from build123d import *

# Parameters (mm, degrees)
F0_W     = 57.15
F0_H     = 38.1
F1_DEPTH = 6.35
F3_DEPTH = 19.05
F5_DEPTH = 25.401
F6_R     = 6.35
F7_SIZE  = 1.27


with BuildPart() as f1:
    # F0 (on Front) → F1 (new body)
    with BuildSketch(Plane.XZ):
        Rectangle(F0_W, F0_H)
    extrude(amount=-F1_DEPTH)

    # F2 (on face) → F3 (join)
    with BuildSketch(Plane.XZ):
        Polygon((-19.05, 19.05), (-25.4, 19.05), (-25.4, 0), (-15.875, 0), (-15.875, -19.05), (15.875, -19.05), (15.875, 0), (25.4, 0), (25.4, 19.05), (19.05, 19.05), (19.05, 6.35), (-19.05, 6.35), align=None)
    extrude(amount=F3_DEPTH)

    # F4 (on face) → F5 (cut, through all)
    with BuildSketch(Plane.XZ.offset(19.05)):
        with BuildLine():
            Line((-11.828537, -19.05), (13.571463, -19.05))
            ThreePointArc((13.571463, -19.05), (0.871463, -6.35), (-11.828537, -19.05))
        make_face()
    extrude(amount=-F5_DEPTH, mode=Mode.SUBTRACT)

    # F6
    f6_edges = [f1.edges().sort_by_distance(p)[0] for p in [
        (-28.575, 3.175, -19.05),
        (28.575, 3.175, -19.05),
        (15.875, -9.525, 0),
        (-15.875, -9.525, 0),
    ]]
    fillet(f6_edges, radius=F6_R)

    # F7
    f7_edges = [f1.edges().sort_by_distance(p)[0] for p in [
        (0.871463, -19.05, -6.35),
        (0, -19.05, 6.35),
        (-19.05, -19.05, 12.7),
        (19.05, -19.05, 12.7),
    ]]
    chamfer(f7_edges, length=F7_SIZE)


solid = f1.part
Geometry check sheet. Reference: the model listing, model coordinates, mm. A direction names the side the tool comes from. Round coordinates to 2 decimals unless told otherwise and drop trailing zeros. Loops run counter-clockwise (first coordinate to the right, second up) from the corner with the lowest first, then second, coordinate; pieces in that order, holes last.
Item 1: Thickness scan on line 1 (X direction, y = -2, z = 9); line 2 (Y direction, x = 18, z = -4.5); line 3 (X direction, y = -11, z = 1). Record the ranges inside material, lowest first.
Item 2: Cross-section at D-D on y = 4.5. Record the boundary of the cut face in (x, z) (3 decimals).
Item 3: Cross-section at B-B on y = -9.5. Record the boundary of the cut face in (x, z) (3 decimals), then the cut area to 3 significant figures.
Item 4: Access from +Z, -Z, +X, -X, +Y, -Y to the whole of each face (thin tool, end or side, straight path). Record for faces 5 (the flat face through (24, -9, 0)), 6 (the flat face through (25.4, -9, 9)), 7 (the flat face through (-19.68, -18.41, 11.97)), 8 (the flat face through (-15.875, -9, -13)).
Item 5: Cross-section at A-A on x = -14. Record the boundary of the cut face in (y, z).
Item 6: Cross-section at C-C on z = 14.5. Record the boundary of the cut face in (x, y) (3 decimals).
Item 7: Gauge pin test, flat ends, axial feed: pin 1 (1 mm diameter, centred on y = -14.5, z = -6.5, fed in from -X); pin 2 (15 mm diameter, centred on y = -12, z = 5.5, fed in from -X); pin 3 (10 mm diameter, centred on y = -10, z = 12.5, fed in from +X). Record the tip position at first contact, or that the pin passes through.
Item 8: Mould release check, pull along X, two halves, no side actions. Record for faces 1 (the flat face through (-28.575, 3, 3)), 2 (the flat face through (15, -1, -19.05)), 3 (the flat face through (15.875, -9, -13)), 4 (the flat face through (19.05, -9, 13)): pulls with the +X half, pulls with the -X half, needs draft (parallel to the pull), parting line crosses it, or undercut.
Answer sheet:
1. line 1: x = -25.4 to -19.05, 19.05 to 25.4
1. line 2: y = 0 to 6.35
1. line 3: x = -25.4 to 25.4
2. outline: (-28.575, -12.7) arc R6.35 ccw to (-22.225, -19.05) - (-11.829, -19.05) arc R12.7 cw to (13.571, -19.05) - (22.225, -19.05) arc R6.35 ccw to (28.575, -12.7) - (28.575, 19.05) - (-28.575, 19.05) - close
3. outline: (-25.4, 0) - (-22.225, 0) arc R6.35 cw to (-15.875, -6.35) - (-15.875, -19.05) - (-11.829, -19.05) arc R12.7 cw to (13.571, -19.05) - (15.875, -19.05) - (15.875, -6.35) arc R6.35 cw to (22.225, 0) - (25.4, 0) - (25.4, 19.05) - (19.05, 19.05) - (19.05, 6.35) - (-19.05, 6.35) - (-19.05, 19.05) - (-25.4, 19.05) - close
3. area: 853 mm2
4. face 5: -Z, +X, -Y
4. face 6: +Z, -Z, +X, -Y
4. face 7: +Z, -Y
4. face 8: -Z, -X, -Y
5. outline: (-19.05, -19.05) - (6.35, -19.05) - (6.35, 19.05) - (0, 19.05) - (0, 6.35) - (-17.78, 6.35) - (-19.05, 5.08) - close
6. outline: (-28.575, 0) - (-25.4, 0) - (-25.4, -19.05) - (-20.32, -19.05) - (-19.05, -17.78) - (-19.05, 0) - (19.05, 0) - (19.05, -17.78) - (20.32, -19.05) - (25.4, -19.05) - (25.4, 0) - (28.575, 0) - (28.575, 6.35) - (-28.575, 6.35) - close
7. pin 1: stops at x = -15.88
7. pin 2: stops at x = -25.4
7. pin 3: stops at x = 25.4
8. face 1: pulls with the -X half
8. face 2: needs draft
8. face 3: pulls with the +X half
8. face 4: undercut
